Model file for the job. Use its own axes, mm. A direction names the side the tool comes from. Round coordinates to 2 decimals unless told otherwise and drop trailing zeros. Order: outer loops, then holes, each group sorted by start corner. A loop starts at its lowest first (then second) coordinate and runs counter-clockwise, first axis right, second up. Notation, with made-up numbers: (-20, 79) -> (15, 79) arc R35 cw to (15, 115) -> close; hole circle Ø7 at (32, 57). An arc over 180 degrees is marked (long way). Put each result on its own line as item: value. Start each with the question number.
Q1. Probe L1, parallel to X at y = 1.4, z = 7.5; L2, parallel to Z at x = 40, y = 1.45; L3, parallel to X at y = 12.75, z = 2.5. List the from-to ranges inside material, lowest first.
Q2. Cut at C-C, the plane x = -4.5. List the corners of the cut face in (y, z).
Q3. Flat gauge pins, fed straight in: P1, Ø3, axis at x = 55.5, z = 2.5, coming from the -Y side; P2, Ø2, axis at x = 40, z = 7.5, coming from the +Y side; P3, Ø1, axis at y = 10, z = 9.5, coming from the -X side. Where does each tip first touch, or does it go through?
Q4. Cut at D-D, the plane y = 6. List the corners of the cut face in (x, z).
Q5. Cut at B-B, the plane z = 2.5. List the corners of the cut face in (x, y).
Q6. 3-axis set-ups, long thin cutter, end or side, ignore diameter. For faces 4 (the face through (56.74, 13.01, 12.34)), 5 (the face through (54, 14, 7)), 6 (the face through (25, 2, 7)), 7 (the face through (-2, 6, 8)), 8 (the face through (53, 6, 8)): which of +Z, -Z, +X, -X, +Y, -Y reach the whole face in a straight line?
Q7. Pull direction X, two halves, no side cores. Call faces 1 (the face through (58, 13, 8)), 2 (the face through (0, 8, 8)), 3 (the face through (25, 0, 7)): released by +X, released by -X, zero draft, split by the parting line, or undercut.
Q8. Cut at A-A, the plane y = 13. List the corners of the cut face in (x, z).
from build123d import *

# Parameters (mm, degrees)
SKETCH_1_W      = 50
SKETCH_1_H      = 15
SKETCH_1_R      = 0.8
EXTRUDE_2_DEPTH = 2
SKETCH_1_5_W    = 2
SKETCH_1_5_H    = 15
SKETCH_1_5_W_2  = 3
EXTRUDE_3_DEPTH = 14
EXTRUDE_START   = 14
SKETCH_1_6_R    = 1.25
EXTRUDE_4_DEPTH = 2


with BuildPart() as part:
    # 草图1 → 凸台-拉伸2 (new body)
    with BuildSketch(Plane(origin=(0, 0, 0), x_dir=(1, 0, 0), z_dir=(0, 1, 0))):
        with Locations((25, -7.5)):
            Rectangle(SKETCH_1_W, SKETCH_1_H)
        with Locations(Location((10, -7.5, 0), (0, 0, 270))):
            Circle(SKETCH_1_R, mode=Mode.SUBTRACT)
        with Locations(Location((40, -7.5, 0), (0, 0, 270))):
            Circle(SKETCH_1_R, mode=Mode.SUBTRACT)
    extrude(amount=EXTRUDE_2_DEPTH)

    # 草图1<5> → 凸台-拉伸3 (add)
    with BuildSketch(Plane(origin=(0, 0, 0), x_dir=(1, 0, 0), z_dir=(0, 1, 0))):
        with Locations((-1, -7.5)):
            Rectangle(SKETCH_1_5_W, SKETCH_1_5_H)
        with Locations((51.5, -7.5)):
            Rectangle(SKETCH_1_5_W_2, SKETCH_1_5_H)
    extrude(amount=EXTRUDE_3_DEPTH)

    # 草图1<6> → 凸台-拉伸4 (add)
    # profile 1 of 2: a face of its own
    with BuildSketch(Plane(origin=(0, 0, 0), x_dir=(1, 0, 0), z_dir=(0, 1, 0)).offset(EXTRUDE_START)):
        Polygon((-2, 0), (-4.5, 0), (-7, 0), (-7, -15), (-4.5, -15), (-2, -15), align=None)
        with Locations(Location((-4.5, -12.5, 0), (0, 0, 270))):
            Circle(SKETCH_1_6_R, mode=Mode.SUBTRACT)
        with Locations(Location((-4.5, -2.5, 0), (0, 0, 270))):
            Circle(SKETCH_1_6_R, mode=Mode.SUBTRACT)
    # profile 2 of 2: a face of its own
    with BuildSketch(Plane(origin=(0, 0, 0), x_dir=(1, 0, 0), z_dir=(0, 1, 0)).offset(EXTRUDE_START)):
        Polygon((55.5, 0), (53, 0), (53, -15), (58, -15), (58, 0), align=None)
        with Locations(Location((55.5, -12.5, 0), (0, 0, 270))):
            Circle(SKETCH_1_6_R, mode=Mode.SUBTRACT)
        with Locations(Location((55.5, -2.5, 0), (0, 0, 270))):
            Circle(SKETCH_1_6_R, mode=Mode.SUBTRACT)
    extrude(amount=-EXTRUDE_4_DEPTH)


solid = part.part
Ans:
1. L1: x = -2 to 9.2, 10.8 to 39.2, 40.8 to 53
1. L2: z = 0 to 6.7, 8.3 to 15
1. L3: x = -7 to -5.75, -3.25 to 0, 50 to 54.25, 56.75 to 58
2. outline: (12, 0) -> (14, 0) -> (14, 1.25) -> (12, 1.25) -> close; (12, 3.75) -> (14, 3.75) -> (14, 11.25) -> (12, 11.25) -> close; (12, 13.75) -> (14, 13.75) -> (14, 15) -> (12, 15) -> close
3. P1: stops at y = 12
3. P2: stops at y = 2
3. P3: stops at x = -2
4. outline: (-2, 0) -> (0, 0) -> (0, 15) -> (-2, 15) -> close; (50, 0) -> (53, 0) -> (53, 15) -> (50, 15) -> close
5. outline: (-7, 12) -> (-5.75, 12) -> (-5.75, 14) -> (-7, 14) -> close; (-3.25, 12) -> (-2, 12) -> (-2, 0) -> (53, 0) -> (53, 12) -> (54.25, 12) -> (54.25, 14) -> (50, 14) -> (50, 2) -> (0, 2) -> (0, 14) -> (-3.25, 14) -> close; (56.75, 12) -> (58, 12) -> (58, 14) -> (56.75, 14) -> close
6. face 4: +Y, -Y
6. face 5: +Z, -Z, +X, -X, +Y
6. face 6: +Z, -Z, +Y
6. face 7: +Z, -Z, -X, -Y
6. face 8: +Z, -Z, +X, -Y
7. face 1: released by +X
7. face 2: undercut
7. face 3: zero draft
8. outline: (-7, 0) -> (0, 0) -> (0, 15) -> (-7, 15) -> close; (50, 0) -> (58, 0) -> (58, 15) -> (50, 15) -> close; hole circle Ø2.5 at (-4.5, 2.5); hole circle Ø2.5 at (-4.5, 12.5); hole circle Ø2.5 at (55.5, 2.5); hole circle Ø2.5 at (55.5, 12.5)
